from build123d import *

# Parameters (mm, degrees)
SKETCH_1_W          = 42
SKETCH_1_H          = 42
EXTRUDE_1_DEPTH     = 7
SKETCH_2_R          = 17.5
CUT_EXTRUDE_1_DEPTH = 31.512292605
SKETCH_3_R          = 18.5
CUT_EXTRUDE_2_DEPTH = 4
SKETCH_4_R          = 19
CUT_EXTRUDE_3_DEPTH = 2
FILLET_1_R          = 4
SKETCH_5_R          = 1.55
CUT_EXTRUDE_4_DEPTH = 31.512292605
SKETCH_7_R          = 1.05
CUT_EXTRUDE_5_DEPTH = 31.512292605
SKETCH_8_R          = 2
CUT_EXTRUDE_6_DEPTH = 3


with BuildPart() as part:
    # 草图1 → 凸台-拉伸1 (new body)
    with BuildSketch(Plane.XY):
        Rectangle(SKETCH_1_W, SKETCH_1_H)
    extrude(amount=EXTRUDE_1_DEPTH)

    # 草图2 → 切除-拉伸1 (cut, through all)
    with BuildSketch(Plane.XY.offset(7)):
        Circle(SKETCH_2_R)
    extrude(amount=-CUT_EXTRUDE_1_DEPTH, mode=Mode.SUBTRACT)

    # 草图3 → 切除-拉伸2 (cut)
    with BuildSketch(Plane.XY.offset(7)):
        Circle(SKETCH_3_R)
    extrude(amount=-CUT_EXTRUDE_2_DEPTH, mode=Mode.SUBTRACT)

    # 草图4 → 切除-拉伸3 (cut)
    with BuildSketch(Plane.XY.offset(7)):
        Circle(SKETCH_4_R)
    extrude(amount=-CUT_EXTRUDE_3_DEPTH, mode=Mode.SUBTRACT)

    # 圆角1
    fillet_1_edges = [part.edges().sort_by_distance(p)[0] for p in [
        (21, -21, 3.5),
        (-21, -21, 3.5),
        (-21, 21, 3.5),
        (21, 21, 3.5),
    ]]
    fillet(fillet_1_edges, radius=FILLET_1_R)

    # 草图5 → 切除-拉伸4 (cut, through all)
    with BuildSketch(Plane.XY.offset(7)):
        with Locations((-16.970562748, 16.970562748)):
            Circle(SKETCH_5_R)
        with Locations((16.970562748, 16.970562748)):
            Circle(SKETCH_5_R)
        with Locations((16.970562748, -16.970562748)):
            Circle(SKETCH_5_R)
        with Locations((-16.970562748, -16.970562748)):
            Circle(SKETCH_5_R)
    extrude(amount=-CUT_EXTRUDE_4_DEPTH, mode=Mode.SUBTRACT)

    # 草图7 → 切除-拉伸5 (cut, through all)
    with BuildSketch(Plane(origin=(0, 0, 0), x_dir=(-1, 0, 0), z_dir=(0, 0, -1))):
        with Locations((-18, 12)):
            Circle(SKETCH_7_R)
        with Locations(Location((18, 12, 0), (0, 0, 180))):
            Circle(SKETCH_7_R)
        with Locations((18, -12)):
            Circle(SKETCH_7_R)
        with Locations(Location((-18, -12, 0), (0, 0, 180))):
            Circle(SKETCH_7_R)
    extrude(amount=-CUT_EXTRUDE_5_DEPTH, mode=Mode.SUBTRACT)

    # 草图8 → 切除-拉伸6 (cut)
    with BuildSketch(Plane(origin=(0, 0, 0), x_dir=(-1, 0, 0), z_dir=(0, 0, -1))):
        with Locations((-18, 12)):
            Circle(SKETCH_8_R)
        with Locations(Location((18, 12, 0), (0, 0, 180))):
            Circle(SKETCH_8_R)
        with Locations((18, -12)):
            Circle(SKETCH_8_R)
        with Locations(Location((-18, -12, 0), (0, 0, 180))):
            Circle(SKETCH_8_R)
    extrude(amount=-CUT_EXTRUDE_6_DEPTH, mode=Mode.SUBTRACT)


solid = part.part
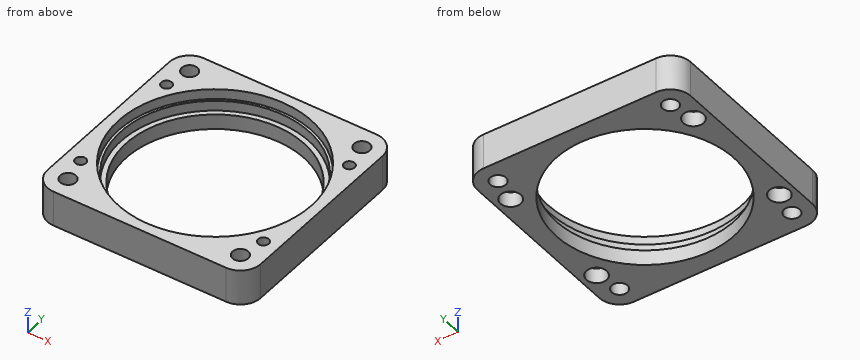
Source: CAD feature listing. Evaluate the final solid. Frame: model axes, mm. Coordinates: 2 decimals unless noted, no trailing zeros. Order: outer loops, then holes, each group sorted by start corner. A loop starts at its lowest first (then second) coordinate and runs counter-clockwise, first axis right, second up. Notation, with made-up numbers: M -31,-12.5 L 1,-12.5 A27 ccw 1,3.5 Z; hole C 34.5,89 d6. An arc over 180 degrees is marked long. Write each question's results on one line, items separated by ' | '. Start each with the question number.
1. Material intervals for L1, parallel to Y at x = -0.5, z = 3.75; L2, parallel to Y at x = 0, z = 5.45; L3, parallel to X at y = -16, z = 6.75, sorted ascending.
2. Pin query (flat end, axial travel): pin 1 (2.5 mm diameter, centred on x = -18, y = -12, fed in from -Z); pin 2 (18.5 mm diameter, centred on x = -3, y = 8, fed in from +Z). Return the tip coordinate at first contact, or that it passes through.
3. Section C-C, the plane y = -12. State how many separate pieces and enclosed holes the cut face has, then the cut area to 3 significant figures.
4. Section A-A, the plane y = 0. Return the cut outline in (x, z), then the cut area to 3 significant figures.
Solution:
1) L1: -21 to -18.49, 18.49 to 21 | L2: -21 to -19, 19 to 21 | L3: -21 to -18.18, -15.76 to -10.25, 10.25 to 15.76, 18.18 to 21
2) pin 1: z = 3 | pin 2: z = 3
3) separate pieces: 4 | enclosed holes: 0 | area: 61.5 mm²
4) outline: M -21,0 L -17.5,0 L -17.5,3 L -18.5,3 L -18.5,5 L -19,5 L -19,7 L -21,7 Z; M 17.5,0 L 21,0 L 21,7 L 19,7 L 19,5 L 18.5,5 L 18.5,3 L 17.5,3 Z | area: 39.0 mm²
